Input: dimensioned drawing with shaded views. Units: mm. Origin: part minimum x, y, z. Give positions to 0.01 mm unless a question says otherwise; leave off trailing zeros. Write each loop counter-clockwise with the first axis right and the second up, starting at its lowest first coordinate (ties: lowest second). Pieces come first, ordered by that corner, then holes. Notation, with made-up numbers: (34, 40.5) - (46, 40.5) arc R32 cw to (46, 66.5) - close; hole circle Ø2 at (-24, -6.75). An arc over 180 degrees is marked (long way). Answer as CSV lines item,"result".
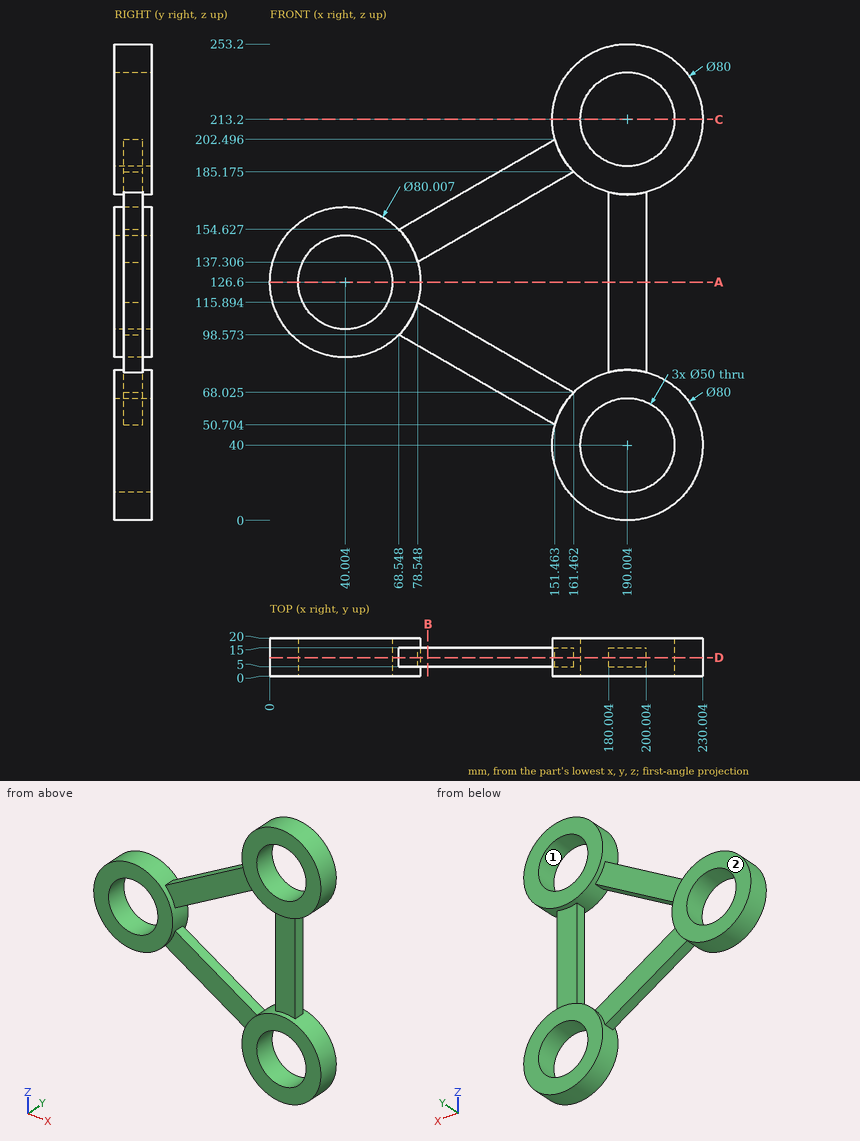
Item 1: Mould query, pull axis Z, two halves, no side actions, for the marked faces 1 and 2. Classes: +Z half, -Z half, draft (parallel to the pull), parting line (faces both ways), or undercut.
The answers:
face 1,"undercut"
face 2,"draft"
Item 2: Cut plane D-D on y = 9.75. Return the cut outline in (x, z) (1 decimal), plus the area to 3 significant figures.
The answers:
outline,"(68.5, 98.6) - (151.5, 50.7) arc R40 ccw (long way) to (200, 78.7) - (200, 174.5) arc R40 ccw (long way) to (151.5, 202.5) - (68.5, 154.6) arc R40 ccw (long way) to start; hole circle Ø50 at (40, 126.6); hole (78.5, 115.9) - (161.5, 68) arc R40 cw to (180, 78.7) - (180, 174.5) arc R40 cw to (161.5, 185.2) - (78.5, 137.3) arc R40 cw to start; hole circle Ø50 at (190, 40); hole circle Ø50 at (190, 213.2)"
area,"14,800 mm²"
Item 3: Contact query for flat-ended pins moving along their axis: pin 1 (8 mm diameter, centred on y = 10, z = 124, fed in from +X); pin 2 (11 mm diameter, centred on y = 10.5, z = 103.5, fed in from -X); pin 3 (16 mm diameter, centred on x = 189.5, z = 147.5, fed in from -Y). Output: stop coordinate, or through.
The answers:
pin 1,"x = 200"
pin 2,"x = 4.08"
pin 3,"y = 5"
Item 4: Cut plane B-B on x = 84. Return the cut outline in (y, z).
The answers:
outline,"(5, 89.65) - (15, 89.65) - (15, 112.75) - (5, 112.75) - close; (5, 140.45) - (15, 140.45) - (15, 163.55) - (5, 163.55) - close"
Item 5: Cut plane A-A on z = 126.6. Return the cut outline in (x, y), plus the area to 3 significant figures.
The answers:
outline,"(0, 0) - (15, 0) - (15, 20) - (0, 20) - close; (65, 0) - (80.01, 0) - (80.01, 20) - (65, 20) - close; (180, 5) - (200, 5) - (200, 15) - (180, 15) - close"
area,"800 mm²"
Item 6: Cut plane C-C on z = 213.2. Return the cut outline in (x, y).
The answers:
outline,"(150, 0) - (165, 0) - (165, 20) - (150, 20) - close; (215, 0) - (230, 0) - (230, 20) - (215, 20) - close"
Item 7: Ray query, line 1 (X direction, y = 14, z = 126.6); line 2 (X direction, y = 14.5, z = 213.2); line 3 (X direction, y = 17, z = 215) (1 decimal). Return the intervals inside material, ascending. Write a range as from..to.
The answers:
line 1,"0..15, 65..80.01, 180..200"
line 2,"150..165, 215..230"
line 3,"150..165.1, 214.9..230"
